Design review of the part shown in the three views and the two pictorial views. Dimensions are in mm from the part's minimum x, y and z. Give positions to 0.01 mm unless a question says otherwise; leave off trailing zeros. Use CSV: the item, a comma, the result in double quotes. Start each with the question number.
Item 1: The part is to be moulded in two halves that separate along Z. For the marked faces 1, 2 and 3, say which applies: +Z half, -Z half, draft (parallel to the pull), parting line (faces both ways), or undercut.
Item 2: Clearance check with flat-ended pins moving along their axes: pin 1 (4 mm diameter, centred on x = 10, z = 10, fed in from +Y); pin 2 (2 mm diameter, centred on x = 2.5, y = 17.5, fed in from -Z); pin 3 (4 mm diameter, centred on x = 10.5, z = 11.5, fed in from -Y); pin 4 (5 mm diameter, centred on x = 13.5, y = 20.5, fed in from -Z). State where each tip first meets the part, or that it passes through.
Item 3: Wall thickness on line 1 along Z through (x, y) = (10, 21.3); line 2 along Z through (x, y) = (10, 10.5); line 3 along Y through (x, z) = (5.5, 1.5): over which ranges is each line inside the solid? List them lowest first. Write a range as from..to.
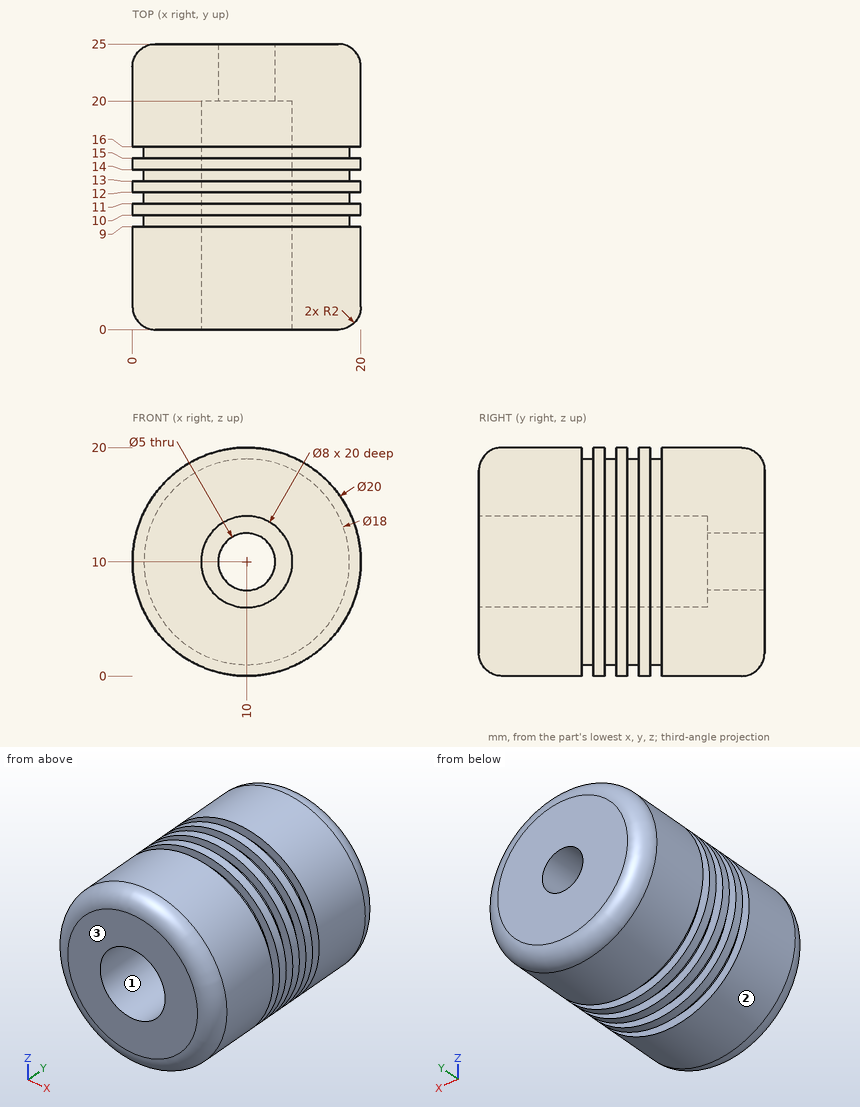
Results found:
1,face 1,"undercut"
1,face 2,"parting line"
1,face 3,"draft"
2,pin 1,"through"
2,pin 2,"z = 2.4"
2,pin 3,"y = 20"
2,pin 4,"z = 0.05"
3,line 1,"0..7.5, 12.5..20"
3,line 2,"0..6, 14..20"
3,line 3,"0.82..9, 10..11, 12..13, 14..15, 16..24.18"
